Here's how the part is built. I have some questions about the finished solid (model axes, mm). Face numbers are marked on the shaded views. A direction names the side the tool comes from. Round coordinates to 2 decimals unless told otherwise and drop trailing zeros. Write each loop counter-clockwise with the first axis right and the second up, starting at its lowest first coordinate (ties: lowest second). Pieces come first, ordered by that corner, then holes. Notation, with made-up numbers: (24.5, -13.75) -> (51.5, -13.75) arc R15 ccw to (51.5, 11.25) -> close; hole circle Ø5 at (20.25, -9). An arc over 180 degrees is marked (long way). Put each result on its own line as item: value. Start each with the question number.
1) If I drill on line 1 along X through (y, z) = (-30, -58); line 2 along X through (y, z) = (-36, -34); line 3 along Z through (x, y) = (98, -22.5), over which ranges is the centre line in solid material (lowest first)? Write a range as [from, to].
2) I want a section at B-B, the plane x = 95. List the corners of the cut face in (y, z) for me.
3) Which directions (+Z, -Z, +X, -X, +Y, -Y) give clear straight access to the entire face, cutting with the end or side of a thin tool? Please do the marked faces 4, 5 and 6.
4) Will these pins go through, and if not, where does the flat tip stop? P1, Ø1.5, axis at x = -13, z = 31, coming from the -Y side; P2, Ø12, axis at x = -50, z = -39, coming from the +Y side.
5) I want a section at C-C, the plane y = -5.5. List the corners of the cut face in (x, z) for me, then the cut area to 3 significant figures.
6) We'd pull the mould along X, two halves only. Please class the marked faces 1, 2 and 3: released by +X, released by -X, zero draft, split by the parting line, or undercut.
7) I want a section at A-A, the plane y = -30. List the corners of the cut face in (x, z) for me.
8) I want a section at D-D, the plane x = -60. List the corners of the cut face in (y, z) for me.
from build123d import *

# Parameters (mm, degrees)
F0_W     = 260
F0_H     = 130
F1_DEPTH = 50
F2_R     = 50
F3_DEPTH = 10
F4_W     = 240
F4_H     = 110
F5_DEPTH = 30
F6_R     = 3.5
F7_DEPTH = 50


with BuildPart() as f1:
    # F0 (on Front) → F1 (new body)
    with BuildSketch(Plane.XZ):
        Rectangle(F0_W, F0_H)
    extrude(amount=F1_DEPTH)

    # F2 (on face) → F3 (cut)
    with BuildSketch(Plane(origin=(0, 0, 0), x_dir=(-1, 0, 0), z_dir=(0, 1, 0))):
        with Locations((60, 0)):
            Circle(F2_R)
        with Locations((-60, 0)):
            Circle(F2_R)
    extrude(amount=-F3_DEPTH, mode=Mode.SUBTRACT)

    # F4 (on face) → F5 (cut)
    with BuildSketch(Plane.XZ.offset(50)):
        Rectangle(F4_W, F4_H)
    extrude(amount=-F5_DEPTH, mode=Mode.SUBTRACT)

    # F6 (on face) → F7 (cut)
    with BuildSketch(Plane(origin=(0, 0, -65), x_dir=(1, 0, 0), z_dir=(0, 0, -1))):
        with Locations((95, 30)):
            Circle(F6_R)
        with Locations((-95, 30)):
            Circle(F6_R)
    extrude(amount=-F7_DEPTH, mode=Mode.SUBTRACT)


solid = f1.part
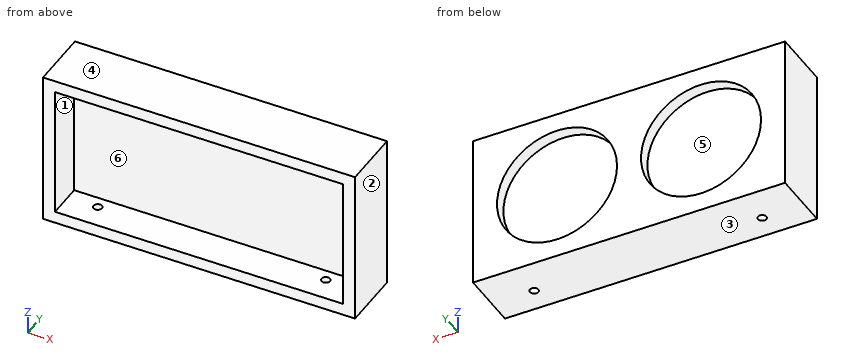
Findings:
1. line 1: x = [-130, -98.5], [-91.5, 91.5], [98.5, 130]
1. line 2: x = [-130, -120], [120, 130]
1. line 3: z = [-65, -55], [55, 65]
2. outline: (-50, -65) -> (-33.5, -65) -> (-33.5, -55) -> (-50, -55) -> close; (-50, 55) -> (-20, 55) -> (-20, -55) -> (-26.5, -55) -> (-26.5, -65) -> (0, -65) -> (0, -35.71) -> (-10, -35.71) -> (-10, 35.71) -> (0, 35.71) -> (0, 65) -> (-50, 65) -> close
3. face 4: +Z, +X, -X, +Y, -Y
3. face 5: +Y
3. face 6: -Y
4. P1: stops at y = -20
4. P2: stops at y = -10
5. outline: (-130, -65) -> (130, -65) -> (130, 65) -> (-130, 65) -> close; hole circle Ø100 at (-60, 0); hole circle Ø100 at (60, 0)
5. area: 18,100 mm2
6. face 1: undercut
6. face 2: released by +X
6. face 3: zero draft
7. outline: (-130, -65) -> (-98.5, -65) -> (-98.5, -55) -> (-120, -55) -> (-120, 55) -> (120, 55) -> (120, -55) -> (98.5, -55) -> (98.5, -65) -> (130, -65) -> (130, 65) -> (-130, 65) -> close; (-91.5, -65) -> (91.5, -65) -> (91.5, -55) -> (-91.5, -55) -> close
8. outline: (-50, -65) -> (0, -65) -> (0, -50) -> (-10, -50) -> (-10, 50) -> (0, 50) -> (0, 65) -> (-50, 65) -> (-50, 55) -> (-20, 55) -> (-20, -55) -> (-50, -55) -> close
